CAD build for the part. Positions are in the model's coordinates, mm. A direction names the side the tool comes from. Give positions to 0.01 mm unless a question says otherwise; leave off trailing zeros. Write each loop counter-clockwise with the first axis right and the second up, starting at its lowest first coordinate (ties: lowest second). Pieces come first, ordered by that corner, then holes. Notation, with made-up numbers: (49.25, 6) - (62.25, 6) arc R28 ccw to (62.25, 31) - close; hole circle Ø8 at (69.25, 89). An arc over 180 degrees is marked (long way). Write item = value, one per line. Start each with the question number.
```python
from build123d import *

# Parameters (mm, degrees)
SKETCH1_W                      = 45
SKETCH1_H                      = 12
BOSS_EXTRUDE1_DEPTH            = 3
SKETCH2_W                      = 3
SKETCH2_H                      = 12
BOSS_EXTRUDE2_DEPTH            = 20
BOSS_EXTRUDE3_DEPTH            = 12
CUT_EXTRUDE3_REACH             = 70.4
SKETCH4_W                      = 32.230769231
SKETCH4_H                      = 9
CUT_EXTRUDE4_REACH             = 70.4
SKETCH5_W                      = 30.769230769
SKETCH5_H                      = 9
CUT_EXTRUDE4_DIRECTION_2_REACH = 70.4
BOSS_EXTRUDE6_DEPTH            = 3
CHAMFER4_SIZE                  = 3
CHAMFER5_SIZE                  = 3
SKETCH9_W                      = 15.6
SKETCH9_H                      = 5.40390508
CUT_EXTRUDE5_DEPTH             = 3
SKETCH10_R                     = 1.6
CUT_EXTRUDE6_DEPTH             = 3
FILLET1_R                      = 2
FILLET2_R                      = 2
FILLET3_R                      = 2


with BuildPart() as part:
    # Sketch1 → Boss-Extrude1 (new body)
    with BuildSketch(Plane.XY):
        Rectangle(SKETCH1_W, SKETCH1_H)
    extrude(amount=BOSS_EXTRUDE1_DEPTH)

    # Sketch2 → Boss-Extrude2 (add)
    with BuildSketch(Plane.XY.offset(3)):
        with Locations((-21, 0)):
            Rectangle(SKETCH2_W, SKETCH2_H)
        with Locations((21, 0)):
            Rectangle(SKETCH2_W, SKETCH2_H)
    extrude(amount=BOSS_EXTRUDE2_DEPTH)

    # Sketch3 → Boss-Extrude3 (add)
    with BuildSketch(Plane(origin=(0, 6, 0), x_dir=(1, 0, 0), z_dir=(0, 1, 0))):
        Polygon((-19.5, -23), (0, -33), (19.5, -23), (22.5, -23), (1.5, -33.769230769), (1.5, -63.769230769), (-1.5, -63.769230769), (-1.5, -33.769230769), (-22.5, -23), align=None)
    extrude(amount=-BOSS_EXTRUDE3_DEPTH)

    # Cut-Extrude3: up to this face of the body (flat: up to its plane)
    cut_extrude3_end = Plane(part.part.faces().sort_by_distance((-1.5, 0, 48.769230769))[0])
    # Sketch4 → Cut-Extrude3 (cut, up to the picked face)
    with BuildSketch(Plane(origin=(1.5, 0, 0), x_dir=(0, 0, -1), z_dir=(1, 0, 0)), mode=Mode.PRIVATE) as cut_extrude3_sk1:
        with Locations((-49.884615385, -1.5)):
            Rectangle(SKETCH4_W, SKETCH4_H)
    cut_extrude3_tool1 = split(extrude(cut_extrude3_sk1.sketch, amount=-CUT_EXTRUDE3_REACH, mode=Mode.PRIVATE), bisect_by=cut_extrude3_end, keep=Keep.BOTH, mode=Mode.PRIVATE)
    add(cut_extrude3_tool1.solids().sort_by(Axis((1.5, -1.5, 49.884615), (-1, 0, 0)))[0], mode=Mode.SUBTRACT)

    # Cut-Extrude4: up to this face of the body (flat: up to its plane)
    cut_extrude4_end = Plane(part.part.faces().sort_by_distance((-22.5, 0, 11.5))[0])
    # Sketch5 → Cut-Extrude4 (cut, up to the picked face)
    with BuildSketch(Plane(origin=(1.5, 0, 0), x_dir=(0, 0, -1), z_dir=(1, 0, 0)), mode=Mode.PRIVATE) as cut_extrude4_sk1:
        with Locations((-18.384615385, -1.5)):
            Rectangle(SKETCH5_W, SKETCH5_H)
    cut_extrude4_tool1 = split(extrude(cut_extrude4_sk1.sketch, amount=-CUT_EXTRUDE4_REACH, mode=Mode.PRIVATE), bisect_by=cut_extrude4_end, keep=Keep.BOTH, mode=Mode.PRIVATE)
    add(cut_extrude4_tool1.solids().sort_by(Axis((1.5, -1.5, 18.384615), (-1, 0, 0)))[0], mode=Mode.SUBTRACT)

    # Cut-Extrude4 direction 2: up to this face of the body (flat: up to its plane)
    cut_extrude4_direction_2_end = Plane(part.part.faces().sort_by_distance((22.5, 0, 11.5))[0])
    # Sketch5 → Cut-Extrude4 direction 2 (cut, up to the picked face)
    with BuildSketch(Plane(origin=(1.5, 0, 0), x_dir=(0, 0, -1), z_dir=(1, 0, 0)), mode=Mode.PRIVATE) as cut_extrude4_direction_2_sk1:
        with Locations((-18.384615385, -1.5)):
            Rectangle(SKETCH5_W, SKETCH5_H)
    cut_extrude4_direction_2_tool1 = split(extrude(cut_extrude4_direction_2_sk1.sketch, amount=CUT_EXTRUDE4_DIRECTION_2_REACH, mode=Mode.PRIVATE), bisect_by=cut_extrude4_direction_2_end, keep=Keep.BOTH, mode=Mode.PRIVATE)
    add(cut_extrude4_direction_2_tool1.solids().sort_by(Axis((1.5, -1.5, 18.384615), (1, 0, 0)))[0], mode=Mode.SUBTRACT)

    # Sketch8 → Boss-Extrude6 (add)
    with BuildSketch(Plane.ZY.offset(1.5)):
        Polygon((63.769230769, 0), (92.169230769, 0), (92.169230769, 3), (66.769230769, 3), (66.769230769, 12.7), (92.169230769, 12.7), (92.169230769, 16), (85.741661946, 16), (63.769230769, 16), (63.769230769, 6), (63.769230769, 3), align=None)
    extrude(amount=-BOSS_EXTRUDE6_DEPTH)

    # Chamfer4
    chamfer4_edges = [part.edges().sort_by_distance(p)[0] for p in [
        (0, 16, 63.769230769),
    ]]
    chamfer(chamfer4_edges, length=CHAMFER4_SIZE)

    # Chamfer5
    chamfer5_edges = [part.edges().sort_by_distance(p)[0] for p in [
        (0, 0, 63.769230769),
    ]]
    chamfer(chamfer5_edges, length=CHAMFER5_SIZE - 0.0001)  # a hair under: the kernel refuses the full size

    # Sketch9 → Cut-Extrude5 (cut)
    with BuildSketch(Plane(origin=(0, 0, 0), x_dir=(-1, 0, 0), z_dir=(0, 0, -1))):
        with Locations((0, 6)):
            Rectangle(SKETCH9_W, SKETCH9_H)
    extrude(amount=-CUT_EXTRUDE5_DEPTH, mode=Mode.SUBTRACT)

    # Sketch10 → Cut-Extrude6 (cut)
    with BuildSketch(Plane(origin=(0, 0, 0), x_dir=(-1, 0, 0), z_dir=(0, 0, -1))):
        with Locations((-9.8, 1.29804746)):
            Circle(SKETCH10_R)
        with Locations((9.8, 1.29804746)):
            Circle(SKETCH10_R)
    extrude(amount=-CUT_EXTRUDE6_DEPTH, mode=Mode.SUBTRACT)

    # Fillet1
    fillet1_edges = [part.edges().sort_by_distance(p)[0] for p in [
        (19.5, 4.5, 23),
        (0, 6, 63.769230769),
        (0, 4.5, 33),
        (-19.5, 4.5, 23),
    ]]
    fillet(fillet1_edges, radius=FILLET1_R)

    # Fillet2
    fillet2_edges = [part.edges().sort_by_distance(p)[0] for p in [
        (21, 3, 3),
        (-21, 3, 3),
    ]]
    fillet(fillet2_edges, radius=FILLET2_R)

    # Fillet3
    fillet3_edges = [part.edges().sort_by_distance(p)[0] for p in [
        (-22.5, -6, 1.5),
        (22.5, -6, 1.5),
    ]]
    fillet(fillet3_edges, radius=FILLET3_R)


solid = part.part
```
1. Cut at A-A (z = 80.5). Give the cut face in (x, y), then the cut area to 3 significant figures.
2. Wall check: line 1 along X through (y, z) = (3.25, 20); line 2 along Y through (x, z) = (-9.8, 1.95); line 3 along Z through (x, y) = (14.5, 0). Give the ranges that are in metal, low to high.
3. Pin check, flat tips, straight feed: pin 1 Ø3 at (x, y) = (9.8, 1.3) entering from -Z; pin 2 Ø1.5 at (x, z) = (0.5, 81.5) entering from -Y; pin 3 Ø8 at (y, z) = (7, 61.5) entering from -X; pin 4 Ø2 at (x, y) = (4, 6) entering from +Z. Stop position of each tip, or through.
4. Mould opens along Z. For faces 1 (the flat face through (1.5, 7, 65)), 2 (the cylindrical face through (-19.215, 4.521, 22.808)), 3 (the flat face through (0, 8, 66.769)) say: +Z half, -Z half, draft (parallel to the pull), parting line (faces both ways), or undercut.
5. Cut at C-C (x = 10). Give the cut face in (y, z).
6. Cut at D-D (z = 39). Give the cut face in (x, y).
7. Tool access for faces 4 (the flat face through (0, 3, 80)), 5 (the flat face through (-7.8, 5, 1)), 6 (the flat face through (-1.5, 7, 65)): list every direction of +Z, -Z, +X, -X, +Y, -Y with a clear straight run to the whole face (end or side of a thin tool).
8. Cut at B-B (x = -15.5). Give the cut face in (y, z).
Output:
q1.outline = (-1.5, 0) - (1.5, 0) - (1.5, 3) - (-1.5, 3) - close; (-1.5, 12.7) - (1.5, 12.7) - (1.5, 16) - (-1.5, 16) - close
q1.area = 18.9 mm2
q2.line_1 = -22.5 to -19.5, 19.5 to 22.5
q2.line_2 = -6 to -0.3, 2.9 to 6
q2.line_3 = 0 to 3
q3.pin_1 = through
q3.pin_2 = 0
q3.pin_3 = -1.5
q3.pin_4 = 33
q4.face_1 = draft
q4.face_2 = undercut
q4.face_3 = +Z half
q5.outline = (-6, 0) - (-0.29, 0) - (-0.29, 3) - (-6, 3) - close; (2.89, 0) - (6, 0) - (6, 3) - (2.89, 3) - close; (3, 27.87) - (6, 27.87) - (6, 29.41) - (3, 29.41) - close
q6.outline = (-1.5, 3) - (1.5, 3) - (1.5, 6) - (-1.5, 6) - close
q7.face_4 = +Z, +X, -X
q7.face_5 = -Z, +Y
q7.face_6 = +Z, -X, +Y, -Y
q8.outline = (-6, 0) - (6, 0) - (6, 3) - (-6, 3) - close; (3, 25.05) - (6, 25.05) - (6, 26.59) - (3, 26.59) - close
